from build123d import *

# Parameters (mm, degrees)
BOSS_EXTRU_1_DEPTH      = 400
ESQUISSE3_R             = 2
ENL_V_MAT_EXTRU_2_DEPTH = 402.940294074
ESQUISSE4_R             = 2.5
ENL_V_MAT_EXTRU_3_DEPTH = 10


with BuildPart() as part:
    # Esquisse1 → Boss.-Extru.1 (new body)
    with BuildSketch(Plane.XY):
        Polygon((-1, -1), (-1, 20), (0, 20), (0, 0), (34, 0), (34, -1), align=None)
    extrude(amount=BOSS_EXTRU_1_DEPTH)

    # Esquisse3 → Enlèv. mat.-Extru.2 (cut, through all)
    with BuildSketch(Plane(origin=(0, 0, 0), x_dir=(1, 0, 0), z_dir=(0, 1, 0))):
        with Locations(Location((29, -206.260283716, 0), (0, 0, 270))):
            Circle(ESQUISSE3_R)
        with Locations(Location((29, -159.260283716, 0), (0, 0, 270))):
            Circle(ESQUISSE3_R)
    extrude(amount=-ENL_V_MAT_EXTRU_2_DEPTH, mode=Mode.SUBTRACT)

    # Esquisse4 → Enlèv. mat.-Extru.3 (cut)
    with BuildSketch(Plane.ZY.offset(1)):
        with Locations(Location((15, 13, 0), (0, 0, 270))):
            Circle(ESQUISSE4_R)
        with Locations(Location((385, 13, 0), (0, 0, 270))):
            Circle(ESQUISSE4_R)
    extrude(amount=-ENL_V_MAT_EXTRU_3_DEPTH, mode=Mode.SUBTRACT)


solid = part.part
Part model, mm, in its own coordinate system. Coordinates: 2 decimals unless noted, no trailing zeros. Loops run counter-clockwise (first coordinate to the right, second up) from the corner with the lowest first, then second, coordinate; pieces in that order, holes last. Notation, with made-up numbers: M 17,57 L 42,57 A24 ccw 42,85 Z; hole C 36.5,46.5 d7. An arc over 180 degrees is marked long. Use a Markdown table: item, result. Add a question column.
Q1. Probe L1, parallel to Z at x = -0.2, y = 13; L2, parallel to X at y = 9.5, z = 149.5; L3, parallel to Y at x = -0.7, z = 385. List the from-to ranges inside material, lowest first.
Q2. Mould opens along X. For faces 1 (the flat face through (17, 0, 197)), 2 (the flat face through (-1, 9, 197)), 3 (the flat face through (0, 10, 197)) say: +X half, -X half, draft (parallel to the pull), parting line (faces both ways), or undercut.
Q3. Pin check, flat tips, straight feed: P1, Ø6, axis at y = 6.5, z = 70, coming from the +X side; P2, Ø10, axis at x = 17, z = 315, coming from the +Y side. Stop position of each tip, or through.
Q4. Cut at A-A (z = 126). Write the cut outline in (x, y), and give its area (3 significant figures).
Q5. Cut at B-B (x = 13). Write the cut outline in (y, z), and give its area (3 significant figures).
Worked out:
| question | item | result |
|---|---|---|
| 1 | L1 | z = 0 to 12.5, 17.5 to 382.5, 387.5 to 400 |
| 1 | L2 | x = -1 to 0 |
| 1 | L3 | y = -1 to 10.5, 15.5 to 20 |
| 2 | face 1 | draft |
| 2 | face 2 | -X half |
| 2 | face 3 | +X half |
| 3 | P1 | stops at x = 0 |
| 3 | P2 | stops at y = 0 |
| 4 | outline | M -1,-1 L 34,-1 L 34,0 L 0,0 L 0,20 L -1,20 Z |
| 4 | area | 55.0 mm2 |
| 5 | outline | M -1,0 L 0,0 L 0,400 L -1,400 Z |
| 5 | area | 400 mm2 |
